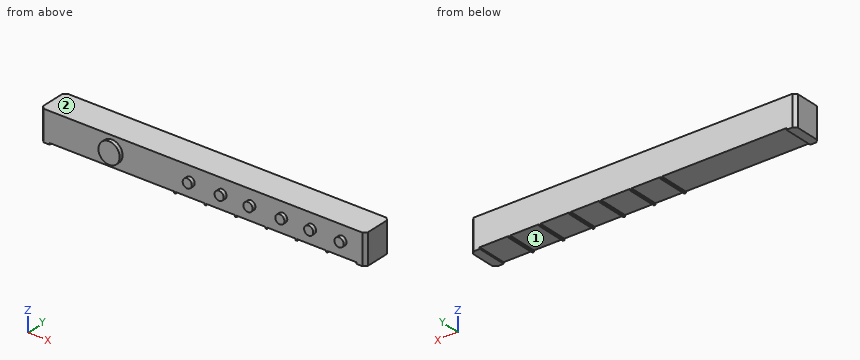
```python
from build123d import *

# Parameters (mm, degrees)
CROQUIS1_W              = 100
CROQUIS1_H              = 100
SALIENTE_EXTRUIR2_DEPTH = 100
CROQUIS2_W              = 410
CROQUIS2_H              = 100
CROQUIS2_W_2            = 95
CORTAR_EXTRUIR2_DEPTH   = 5
CROQUIS3_R              = 15
CROQUIS3_R_2            = 35
SALIENTE_EXTRUIR3_DEPTH = 50


with BuildPart() as part:
    # Croquis1 → Saliente-Extruir2 (new body)
    with BuildSketch(Plane.XY):
        Polygon((793.691747165, 62.128712871), (793.691747165, -37.871287129), (893.691747165, -37.871287129), (923.691747165, -37.871287129), (933.691747165, -27.871287129), (933.691747165, 52.128712871), (923.691747165, 62.128712871), (893.691747165, 62.128712871), align=None)
        with Locations((743.691747165, 12.128712871)):
            Rectangle(CROQUIS1_W, CROQUIS1_H)
        with Locations((643.691747165, 12.128712871)):
            Rectangle(CROQUIS1_W, CROQUIS1_H)
        with Locations((543.691747165, 12.128712871)):
            Rectangle(CROQUIS1_W, CROQUIS1_H)
        with Locations((443.691747165, 12.128712871)):
            Rectangle(CROQUIS1_W, CROQUIS1_H)
        with Locations((343.691747165, 12.128712871)):
            Rectangle(CROQUIS1_W, CROQUIS1_H)
        Polygon((-126.308252835, -37.871287129), (-106.308252835, -37.871287129), (293.691747165, -37.871287129), (293.691747165, 62.128712871), (-106.308252835, 62.128712871), (-126.308252835, 62.128712871), (-136.308252835, 52.128712871), (-136.308252835, -27.871287129), align=None)
    extrude(amount=SALIENTE_EXTRUIR2_DEPTH)

    # Croquis2 → Cortar-Extruir2 (cut)
    with BuildSketch(Plane.XY):
        with Locations((98.691747165, 12.128712871)):
            Rectangle(CROQUIS2_W, CROQUIS2_H)
        with Locations((856.191747165, 12.128712871)):
            Rectangle(CROQUIS2_W_2, CROQUIS2_H)
        with Locations((756.191747165, 12.128712871)):
            Rectangle(CROQUIS2_W_2, CROQUIS2_H)
        with Locations((656.191747165, 12.128712871)):
            Rectangle(CROQUIS2_W_2, CROQUIS2_H)
        with Locations((556.191747165, 12.128712871)):
            Rectangle(CROQUIS2_W_2, CROQUIS2_H)
        with Locations((456.191747165, 12.128712871)):
            Rectangle(CROQUIS2_W_2, CROQUIS2_H)
        with Locations((356.191747165, 12.128712871)):
            Rectangle(CROQUIS2_W_2, CROQUIS2_H)
    extrude(amount=CORTAR_EXTRUIR2_DEPTH, mode=Mode.SUBTRACT)

    # Croquis3 → Saliente-Extruir3 (add)
    with BuildSketch(Plane(origin=(0, 0, 0), x_dir=(1, 0, 0), z_dir=(0, 1, 0))):
        with Locations(Location((856.191747165, -52.5, 0), (0, 0, 270))):
            Circle(CROQUIS3_R)
        with Locations(Location((756.191747165, -52.5, 0), (0, 0, 270))):
            Circle(CROQUIS3_R)
        with Locations(Location((661.191747165, -52.5, 0), (0, 0, 270))):
            Circle(CROQUIS3_R)
        with Locations(Location((556.191747165, -52.5, 0), (0, 0, 270))):
            Circle(CROQUIS3_R)
        with Locations(Location((461.191747165, -52.5, 0), (0, 0, 270))):
            Circle(CROQUIS3_R)
        with Locations(Location((356.191747165, -52.5, 0), (0, 0, 270))):
            Circle(CROQUIS3_R)
        with Locations(Location((98.691747165, -52.5, 0), (0, 0, 270))):
            Circle(CROQUIS3_R_2)
    extrude(amount=-SALIENTE_EXTRUIR3_DEPTH)


solid = part.part
```
Part model, mm, in its own coordinate system. Face numbers are marked on the shaded views. A direction names the side the tool comes from. Round coordinates to 2 decimals unless told otherwise and drop trailing zeros. Write each loop counter-clockwise with the first axis right and the second up, starting at its lowest first coordinate (ties: lowest second). Pieces come first, ordered by that corner, then holes.
Item 1: Probe L1, parallel to Y at x = 273, z = 9; L2, parallel to Z at x = 173, y = 13.5; L3, parallel to X at y = 56, z = 89. List the from-to ranges inside material, lowest first.
Results:
L1: y = -37.87 to 62.13
L2: z = 5 to 100
L3: x = -132.44 to 929.82
Item 2: Drop a flat-ended pin along its axis: pin 1 Ø3 at (x, y) = (464.5, 46) entering from -Z. Give the stop position or say it passes through.
Results:
pin 1: stops at z = 5
Item 3: Which spindle directions (+Z, -Z, +X, -X, +Y, -Y) get a long thin tool onto all of the face, cutting with end or side? Do the marked faces 1 and 2. Say none if no direction does.
Results:
face 1: -Z, +Y, -Y
face 2: +Z, +X, -X, +Y, -Y
Item 4: Cut at B-B, the plane x = 253.5. Give the cut face in (y, z).
Results:
outline: (-37.87, 5) - (62.13, 5) - (62.13, 100) - (-37.87, 100) - close
